Geometry check sheet. Reference: the model listing, model coordinates, mm. Coordinates: 2 decimals unless noted, no trailing zeros. Loops run counter-clockwise (first coordinate to the right, second up) from the corner with the lowest first, then second, coordinate; pieces in that order, holes last. Notation, with made-up numbers: M -20,-33 L 32,-33 A27 cw 32,-9 Z; hole C 22,21.25 d2. An arc over 180 degrees is marked long. Use CSV: the item, a comma, the result in double quotes.
Autodesk Inventor part; units mm, degrees
ref_plane "作業平面1" through (0, 5, 0) normal (0, 1, 0) x (-1, 0, 0)
ref_plane "YZ Plane" through (0, 0, 0) normal (1, 0, 0) x (0, 1, 0)
ref_plane "XY Plane" through (0, 0, 0) normal (0, 0, 1) x (1, 0, 0)
sketch "スケッチ1" plane through (0, 0, 0) normal (0, 0, 1) x (1, 0, 0)
  circle A0 centre (0, 0) radius 5
  dimension "d0" = 10
extrude "押し出し1" add sketch "スケッチ1" along normal blind 137
ref_plane "作業平面1" through (0, 5, 0) normal (0, 1, 0) x (-1, 0, 0)
sketch "スケッチ2" plane through (0, 5, 0) normal (0, 1, 0) x (-1, 0, 0)
  line L0 (5, 0) -> (-5, 0)
  line L1 (5, 137) -> (-5, 137)
  point P0 (0, 0)
  point P1 (0, 3)
  point P2 (0, 134)
  point P3 (0, 114)
  point P4 (0, 38)
  point P5 (0, 69.5)
  point P6 (0, 50)
  dimension "d3" = 3
  dimension "d19" = 3
  dimension "d20" = 23
  dimension "d22" = 99
  dimension "d23" = 44.5
  dimension "d24" = 19.5
hole "穴1" at (0, 5, 3) at (0, 5, 134) at (0, 5, 38) direction (0, -1, 0) diameter 2 end through all
hole "穴2" at (0, 5, 114) direction (0, -1, 0) diameter 4 end through all
sketch "スケッチ4" plane through (0, 0, 0) normal (0, 0, -1) x (-1, 0, 0)
  circle A0 centre (0, 0) radius 5
  circle A1 centre (0, 0) radius 5
extrude "押し出し2" cut sketch "スケッチ4" against normal blind 42
properties part number "light_bar_roller_10" material "アルミニウム 6061-AHC"
1. Release check for a two-part mould opening along X. For faces 1 (the cylindrical face through (-1.08, 4.88, 88.84)), 2 (the flat face through (0, 0, 137)), 3 (the cylindrical face through (0, 0, 133)) record: +X half, -X half, draft (parallel to the pull), parting line (faces both ways), or undercut.
The answers:
face 1,"parting line"
face 2,"draft"
face 3,"undercut"
2. Section check D-D, the plane z = 56.5. Record the cut outline in (x, y).
The answers:
outline,"C 0,0 d10"
3. Section check B-B, the plane y = 0. Record the cut outline in (x, z), plus the area to 3 significant figures.
The answers:
outline,"M -5,42 L 5,42 L 5,137 L -5,137 Z; hole C 0,114 d4; hole C 0,134 d2"
area,"934 mm^2"
4. Section check C-C, the plane z = 134. Record the cut outline in (x, y).
The answers:
outline,"M -1,-4.9 L -1,4.9 A5 ccw Z; M 1,-4.9 A5 ccw 1,4.9 Z"
5. Thickness scan on line 1 (Z direction, x = 0, y = 1.5); line 2 (Z direction, x = 0.75, y = 1.5); line 3 (X direction, y = 0.25, z = 134). Record the ranges inside material, lowest first. Write a range as [from, to].
The answers:
line 1,"[42, 112], [116, 133], [135, 137]"
line 2,"[42, 112.15], [115.85, 133.34], [134.66, 137]"
line 3,"[-4.99, -1], [1, 4.99]"
6. Gauge pin test, flat ends, axial feed: P1, Ø1, axis at y = 2, z = 77.5, coming from the +X side; P2, Ø1.5, axis at y = -2, z = 108, coming from the -X side. Record the tip position at first contact, or that the pin passes through.
The answers:
P1,"x = 4.77"
P2,"x = -4.84"
7. Section check A-A, the plane x = 0. Record the cut outline in (y, z).
The answers:
outline,"M -5,42 L 5,42 L 5,112 L -5,112 Z; M -5,116 L 5,116 L 5,133 L -5,133 Z; M -5,135 L 5,135 L 5,137 L -5,137 Z"
